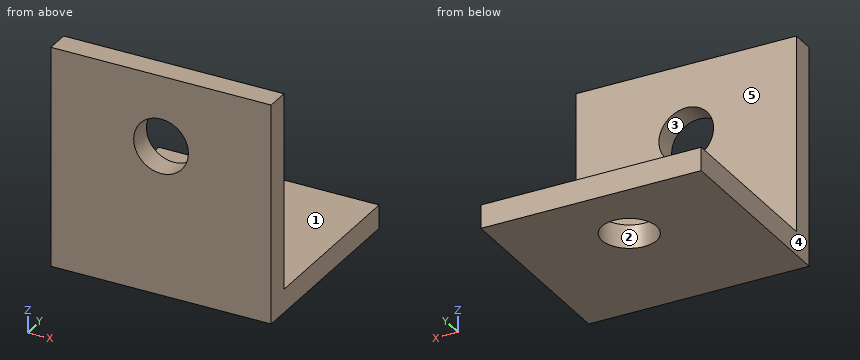
from build123d import *

# Parameters (mm, degrees)
ESBO_O1_W                = 28.2
ESBO_O1_H                = 25.4
RESSALTO_EXTRUS_O1_DEPTH = 3
ESBO_O2_W                = 28.2
ESBO_O2_H                = 3
RESSALTO_EXTRUS_O2_DEPTH = 25.1
ESBO_O3_R                = 3.5
CORTE_EXTRUS_O1_DEPTH    = 3
ESBO_O4_R                = 3.5
CORTE_EXTRUS_O2_DEPTH    = 3


with BuildPart() as part:
    # Esboço1 → Ressalto-extrusão1 (new body)
    with BuildSketch(Plane.XY):
        with Locations((-14.1, 3.482258065)):
            Rectangle(ESBO_O1_W, ESBO_O1_H)
    extrude(amount=RESSALTO_EXTRUS_O1_DEPTH)

    # Esboço2 → Ressalto-extrusão2 (add)
    with BuildSketch(Plane.XY.offset(3)):
        with Locations((-14.1, -7.717741935)):
            Rectangle(ESBO_O2_W, ESBO_O2_H)
    extrude(amount=RESSALTO_EXTRUS_O2_DEPTH)

    # Esboço3 → Corte-extrusão1 (cut)
    with BuildSketch(Plane(origin=(0, -6.217741935, 0), x_dir=(1, 0, 0), z_dir=(0, 1, 0))):
        with Locations(Location((-14.1, -19.1, 0), (0, 0, 270))):
            Circle(ESBO_O3_R)
    extrude(amount=-CORTE_EXTRUS_O1_DEPTH, mode=Mode.SUBTRACT)

    # Esboço4 → Corte-extrusão2 (cut)
    with BuildSketch(Plane.XY.offset(3)):
        with Locations((-14.1, 7.182258065)):
            Circle(ESBO_O4_R)
    extrude(amount=-CORTE_EXTRUS_O2_DEPTH, mode=Mode.SUBTRACT)


solid = part.part
Work out the finished part from the listing and answer in its coordinate system (mm). Face numbers are marked on the shaded views. A direction names the side the tool comes from. Give positions to 0.01 mm unless a question says otherwise; leave off trailing zeros. Write each loop counter-clockwise with the first axis right and the second up, starting at its lowest first coordinate (ties: lowest second). Pieces come first, ordered by that corner, then holes. Notation, with made-up numbers: (28, 25) - (70, 25) arc R26 ccw to (70, 62) - close; hole circle Ø4 at (84.5, 89.25). An arc over 180 degrees is marked (long way). One line per item, written item: value. Start each with the question number.
1. For a pull along Z with two mould halves and no side action, classify the marked faces 1, 2 and 3 as +Z half, -Z half, draft (parallel to the pull), parting line (faces both ways), or undercut.
2. Find section B-B (x = -14.1). Write down the section's boundary in (y, z).
3. Find section A-A (z = 19.1). Write down the section's boundary in (x, y), then the cut area to 3 significant figures.
4. Find section D-D (x = -1.75). Write down the section's boundary in (y, z).
5. Find section C-C (y = 6.5). Write down the section's boundary in (x, z), then the cut area to 3 significant figures.
6. Given pin 1 (10 mm diameter, centred on y = -6, z = 14, fed in from +X); pin 2 (7.5 mm diameter, centred on x = -14, z = 19.5, fed in from +Y); pin 3 (3 mm diameter, centred on x = -9, y = 12, fed in from +Z); pin 4 (5.5 mm diameter, centred on x = -14.1, y = 7.18, fed in from +Z), each flat-ended and moving along its own axis, determine where each tip first touches the part or whether it passes through.
7. Consider probe 1 along X at (y, z) = (-8.1, 19.1); probe 2 along Y at (x, z) = (-14.1, 1.4); probe 3 along Z at (x, y) = (-19.25, 5). Determine where each line is inside the solid, lowest interval first.
8. For the marked faces 4 and 5, determine the directions among +Z, -Z, +X, -X, +Y, -Y from which every point of the face is accessible in a straight line to the end or side of a thin tool.
Geometry results:
1. face 1: +Z half
1. face 2: draft
1. face 3: undercut
2. outline: (-9.22, 0) - (3.68, 0) - (3.68, 3) - (-6.22, 3) - (-6.22, 15.6) - (-9.22, 15.6) - close; (-9.22, 22.6) - (-6.22, 22.6) - (-6.22, 28.1) - (-9.22, 28.1) - close; (10.68, 0) - (16.18, 0) - (16.18, 3) - (10.68, 3) - close
3. outline: (-28.2, -9.22) - (-17.6, -9.22) - (-17.6, -6.22) - (-28.2, -6.22) - close; (-10.6, -9.22) - (0, -9.22) - (0, -6.22) - (-10.6, -6.22) - close
3. area: 63.6 mm2
4. outline: (-9.22, 0) - (16.18, 0) - (16.18, 3) - (-6.22, 3) - (-6.22, 28.1) - (-9.22, 28.1) - close
5. outline: (-28.2, 0) - (-17.53, 0) - (-17.53, 3) - (-28.2, 3) - close; (-10.67, 0) - (0, 0) - (0, 3) - (-10.67, 3) - close
5. area: 64.0 mm2
6. pin 1: x = 0
6. pin 2: y = -6.22
6. pin 3: z = 3
6. pin 4: through
7. probe 1: -28.2 to -17.6, -10.6 to 0
7. probe 2: -9.22 to 3.68, 10.68 to 16.18
7. probe 3: 0 to 3
8. face 4: +Z, -Z, -X, +Y, -Y
8. face 5: +Z, +X, -X, +Y
